from build123d import *

# Parameters (mm, degrees)
SKETCH1_W           = 15
SKETCH1_H           = 15
SKETCH1_W_2         = 11
SKETCH1_H_2         = 11
BOSS_EXTRUDE1_DEPTH = 2
SKETCH5_W           = 2
SKETCH5_H           = 2
BOSS_EXTRUDE2_DEPTH = 11
SKETCH8_W           = 15
SKETCH8_H           = 15
SKETCH8_W_2         = 11
SKETCH8_H_2         = 11
BOSS_EXTRUDE3_DEPTH = 2
BOSS_EXTRUDE4_DEPTH = 2
BOSS_EXTRUDE5_DEPTH = 2
BOSS_EXTRUDE6_DEPTH = 2
SKETCH12_W          = 11
SKETCH12_H          = 11
SKETCH12_R          = 1.5
BOSS_EXTRUDE7_DEPTH = 2
SKETCH13_W          = 11
SKETCH13_H          = 11
SKETCH13_R          = 1.5
BOSS_EXTRUDE8_DEPTH = 2
BOSS_EXTRUDE9_START = -2
SKETCH14_W          = 11
SKETCH14_H          = 11
SKETCH14_R          = 1.5
BOSS_EXTRUDE9_DEPTH = 2


with BuildPart() as part:
    # Sketch1 → Boss-Extrude1 (new body)
    with BuildSketch(Plane(origin=(0, 0, 0), x_dir=(1, 0, 0), z_dir=(0, 1, 0))):
        Rectangle(SKETCH1_W, SKETCH1_H)
        Rectangle(SKETCH1_W_2, SKETCH1_H_2, mode=Mode.SUBTRACT)
    extrude(amount=BOSS_EXTRUDE1_DEPTH)

    # Sketch5 → Boss-Extrude2 (add)
    with BuildSketch(Plane(origin=(0, 2, 0), x_dir=(1, 0, 0), z_dir=(0, 1, 0))):
        with Locations((-6.5, -6.5)):
            Rectangle(SKETCH5_W, SKETCH5_H)
        with Locations((6.5, -6.5)):
            Rectangle(SKETCH5_W, SKETCH5_H)
        with Locations((6.5, 6.5)):
            Rectangle(SKETCH5_W, SKETCH5_H)
        with Locations((-6.5, 6.5)):
            Rectangle(SKETCH5_W, SKETCH5_H)
    extrude(amount=BOSS_EXTRUDE2_DEPTH)

    # Sketch8 → Boss-Extrude3 (add)
    with BuildSketch(Plane(origin=(0, 13, 0), x_dir=(1, 0, 0), z_dir=(0, 1, 0))):
        Rectangle(SKETCH8_W, SKETCH8_H)
        Rectangle(SKETCH8_W_2, SKETCH8_H_2, mode=Mode.SUBTRACT)
    extrude(amount=BOSS_EXTRUDE3_DEPTH)

    # Sketch9 → Boss-Extrude4 (add)
    with BuildSketch(Plane.XZ):
        with BuildLine():
            Line((5.5, 0), (5.5, 5.5))
            Line((5.5, 5.5), (-2e-08, 5.5))
            ThreePointArc((-2e-08, 5.5), (3.88908729, 3.889087304), (5.5, 0))
        make_face()
        with BuildLine():
            ThreePointArc((-5.5, 1.5e-08), (-3.889087298, 3.889087295), (-2e-08, 5.5))
            Line((-2e-08, 5.5), (-5.5, 5.5))
            Line((-5.5, 5.5), (-5.5, 1.5e-08))
        make_face()
        with BuildLine():
            Line((5.5, -5.5), (5.5, 0))
            ThreePointArc((5.5, 0), (3.889087294, -3.889087299), (-7e-09, -5.5))
            Line((-7e-09, -5.5), (5.5, -5.5))
        make_face()
        with BuildLine():
            ThreePointArc((-7e-09, -5.5), (-3.889087305, -3.889087288), (-5.5, 1.5e-08))
            Line((-5.5, 1.5e-08), (-5.5, -5.5))
            Line((-5.5, -5.5), (-7e-09, -5.5))
        make_face()
    extrude(amount=-BOSS_EXTRUDE4_DEPTH)

    # Sketch10 → Boss-Extrude5 (add)
    with BuildSketch(Plane(origin=(0, 0, -7.5), x_dir=(-1, 0, 0), z_dir=(0, 0, -1))):
        with BuildLine():
            Line((-5.5, 13), (-5.5, 7.500000001))
            ThreePointArc((-5.5, 7.500000001), (-3.889087296, 11.389087297), (0, 13))
            Line((0, 13), (-5.5, 13))
        make_face()
        with BuildLine():
            ThreePointArc((0, 13), (3.889087297, 11.389087297), (5.5, 7.5))
            Line((5.5, 7.5), (5.5, 13))
            Line((5.5, 13), (0, 13))
        make_face()
        with BuildLine():
            ThreePointArc((5.5, 7.5), (3.889087297, 3.610912703), (0, 2))
            Line((0, 2), (5.5, 2))
            Line((5.5, 2), (5.5, 7.5))
        make_face()
        with BuildLine():
            Line((-5.5, 7.500000001), (-5.5, 2))
            Line((-5.5, 2), (0, 2))
            ThreePointArc((0, 2), (-3.889087297, 3.610912704), (-5.5, 7.500000001))
        make_face()
    extrude(amount=-BOSS_EXTRUDE5_DEPTH)

    # Sketch11 → Boss-Extrude6 (add)
    with BuildSketch(Plane.ZY.offset(7.5)):
        with BuildLine():
            Line((-5.5, 13), (-5.5, 7.5))
            ThreePointArc((-5.5, 7.5), (-3.88908729, 11.389087303), (1.9e-08, 13))
            Line((1.9e-08, 13), (-5.5, 13))
        make_face()
        with BuildLine():
            ThreePointArc((1.9e-08, 13), (3.889087303, 11.38908729), (5.5, 7.5))
            Line((5.5, 7.5), (5.5, 13))
            Line((5.5, 13), (1.9e-08, 13))
        make_face()
        with BuildLine():
            Line((-5.5, 7.5), (-5.5, 2))
            Line((-5.5, 2), (-7e-09, 2))
            ThreePointArc((-7e-09, 2), (-3.889087299, 3.610912706), (-5.5, 7.5))
        make_face()
        with BuildLine():
            ThreePointArc((5.5, 7.5), (3.889087294, 3.610912701), (-7e-09, 2))
            Line((-7e-09, 2), (5.5, 2))
            Line((5.5, 2), (5.5, 7.5))
        make_face()
    extrude(amount=-BOSS_EXTRUDE6_DEPTH)

    # Sketch12 → Boss-Extrude7 (add)
    with BuildSketch(Plane.XY.offset(7.5)):
        with Locations((0, 7.5)):
            Rectangle(SKETCH12_W, SKETCH12_H)
        with Locations((0, 7.5)):
            Circle(SKETCH12_R, mode=Mode.SUBTRACT)
    extrude(amount=-BOSS_EXTRUDE7_DEPTH)

    # Sketch13 → Boss-Extrude8 (add)
    with BuildSketch(Plane(origin=(0, 15, 0), x_dir=(1, 0, 0), z_dir=(0, 1, 0))):
        Rectangle(SKETCH13_W, SKETCH13_H)
        Circle(SKETCH13_R, mode=Mode.SUBTRACT)
    extrude(amount=-BOSS_EXTRUDE8_DEPTH)

    # Sketch14 → Boss-Extrude9 (add)
    with BuildSketch(Plane(origin=(7.5, 0, 0), x_dir=(0, 0, -1), z_dir=(1, 0, 0)).offset(BOSS_EXTRUDE9_START)):
        with Locations((0, 7.5)):
            Rectangle(SKETCH14_W, SKETCH14_H)
        with Locations((0, 7.5)):
            Circle(SKETCH14_R, mode=Mode.SUBTRACT)
    extrude(amount=BOSS_EXTRUDE9_DEPTH)


solid = part.part
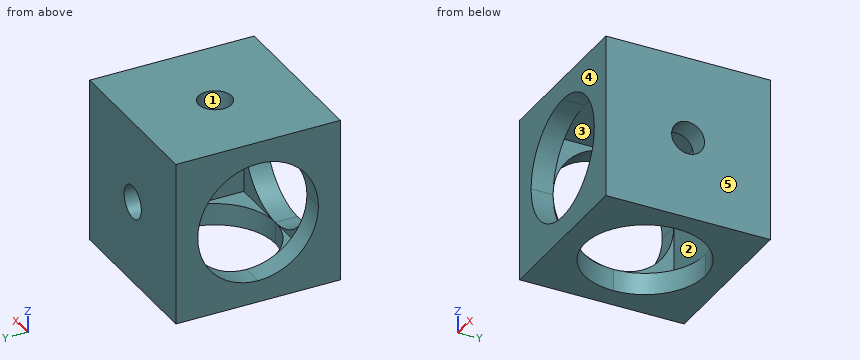
Read the model definition and answer for the solid it produces. Units are mm, in the model's axes. Face numbers are marked on the shaded views. A direction names the side the tool comes from. Give positions to 0.01 mm unless a question says otherwise; leave off trailing zeros. Loops run counter-clockwise (first coordinate to the right, second up) from the corner with the lowest first, then second, coordinate; pieces in that order, holes last. Notation, with made-up numbers: (18, -6) - (76, -6) arc R8 ccw to (76, 7) - close; hole circle Ø9 at (67.25, 42). An arc over 180 degrees is marked (long way). Answer as CSV lines item,"result". Start each with the question number.
1) Determine the mould class of the marked faces 3, 4 and 5 for opening direction X: released by +X, released by -X, zero draft, split by the parting line, or undercut.
2) Which of the six approach directions +Z, -Z, +X, -X, +Y, -Y give full straight-line access (tool end or side, diameter ignored) to the marked faces 1 and 2?
3) Find section B-B (x = -1.25). Write down the section's boundary in (y, z), then the cut area to 3 significant figures.
4) Find section A-A (y = 3). Write down the section's boundary in (x, z).
5) Straight lines are drawn through the part: L1, parallel to Z at x = 0, y = 14.4; L2, parallel to Y at x = -5.25, z = 4.25; L3, parallel to X at y = 5.75, z = 5.25. For each, find the intervals that lie inside material, in ascending order. Write a range as from..to.
6) Find section D-D (y = 13.5). Write down the section's boundary in (x, z).
7) Find section C-C (z = 5.25). Write down the section's boundary in (x, y), then the cut area to 3 significant figures.
8) Each of these flat-tipped pins is pushed along its axis until it touches: pin 1 Ø1 at (x, z) = (-2, -1.5) entering from -Y; pin 2 Ø2.5 at (x, y) = (0, 7.5) entering from -Z. Where does it stop, or does it pass through?
Findings below:
1,face 3,"undercut"
1,face 4,"zero draft"
1,face 5,"released by +X"
2,face 1,"+Z, -Z"
2,face 2,"none"
3,outline,"(0, -7.5) - (2.14, -7.5) - (2.14, -5.5) - (2, -5.5) - (2, -5.36) - (0, -5.36) - close; (0, 5.36) - (2, 5.36) - (2, 5.5) - (6.67, 5.5) - (6.67, 7.5) - (0, 7.5) - close; (8.33, 5.5) - (13, 5.5) - (13, 0.83) - (15, 0.83) - (15, 7.5) - (8.33, 7.5) - close; (12.86, -7.5) - (15, -7.5) - (15, -0.83) - (13, -0.83) - (13, -5.5) - (12.86, -5.5) - close"
3,area,"54.5 mm^2"
4,outline,"(-7.5, -7.5) - (-3.16, -7.5) - (-3.16, -5.5) - (-5.5, -5.5) - (-5.5, -3.16) - (-7.5, -3.16) - close; (-7.5, 3.16) - (-5.5, 3.16) - (-5.5, 5.5) - (5.5, 5.5) - (5.5, -5.5) - (3.16, -5.5) - (3.16, -7.5) - (7.5, -7.5) - (7.5, 7.5) - (-7.5, 7.5) - close"
5,L1,"-7.5..-1.5, 1.5..7.5"
5,L2,"0..2, 13..15"
5,L3,"-7.5..-5.5, 5.5..7.5"
6,outline,"(-7.5, -7.5) - (7.5, -7.5) - (7.5, 7.5) - (-7.5, 7.5) - close; hole circle Ø3 at (0, 0)"
7,outline,"(-7.5, 0) - (-1.64, 0) - (-1.64, 2) - (-5.5, 2) - (-5.5, 5.86) - (-7.5, 5.86) - close; (-7.5, 9.14) - (-5.5, 9.14) - (-5.5, 13) - (5.5, 13) - (5.5, 2) - (1.64, 2) - (1.64, 0) - (7.5, 0) - (7.5, 15) - (-7.5, 15) - close"
7,area,"90.9 mm^2"
8,pin 1,"y = 13"
8,pin 2,"through"
